Geometry: final body of the model. Coordinates: model frame, mm. Face numbers are marked on the shaded views. Coordinates: 2 decimals unless noted, no trailing zeros. Put each result on its own line as item: value.
```python
from build123d import *

# Parameters (mm, degrees)
F0_R     = 2.75
F1_DEPTH = 21
F1_TAPER = -8
F2_DEPTH = 21.0010001


with BuildPart() as f1:
    # F0 (on Top) → F1 (new body)
    with BuildSketch(Plane.XY):
        with BuildLine():
            ThreePointArc((15.2546531369, -7.0046531369), (21.75, 0), (15.2546531369, 7.0046531369))
            Line((15.2546531369, 7.0046531369), (-14.7453468631, 7.0046531369))
            ThreePointArc((-14.7453468631, 7.0046531369), (-21.75, 0), (-14.7453468631, -7.0046531369))
            Line((-14.7453468631, -7.0046531369), (15.2546531369, -7.0046531369))
        make_face()
        with Locations((-14.7453468631, 0)):
            Circle(F0_R, mode=Mode.SUBTRACT)
        with Locations((15.2546531369, 0)):
            Circle(F0_R, mode=Mode.SUBTRACT)
        with Locations((15.2546531369, 0)):
            Circle(F0_R)
        with Locations((-14.7453468631, 0)):
            Circle(F0_R)
    extrude(amount=-F1_DEPTH, taper=F1_TAPER)

    # F0 (on Top) → F2 (cut, through all)
    with BuildSketch(Plane.XY):
        with Locations((15.2546531369, 0)):
            Circle(F0_R)
        with Locations((-14.7453468631, 0)):
            Circle(F0_R)
    extrude(amount=-F2_DEPTH, mode=Mode.SUBTRACT)


solid = f1.part
```
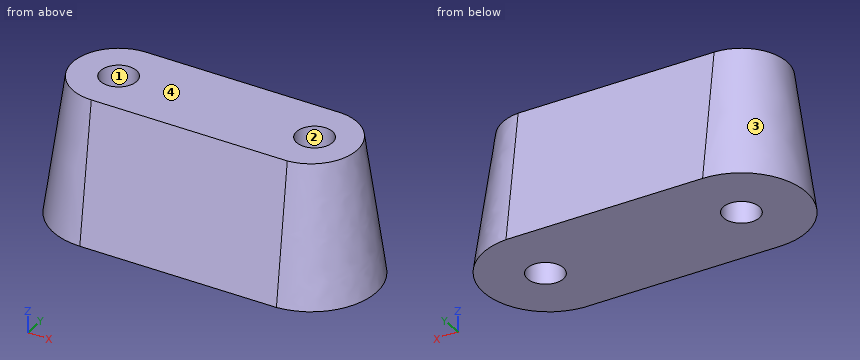
1. Pin query (flat end, axial travel): pin 1 Ø4 at (x, y) = (4.5, 5.5) entering from +Z; pin 2 Ø5 at (x, z) = (-16.5, -4) entering from +Y; pin 3 Ø10 at (y, z) = (3.5, -5.5) entering from -X; pin 4 Ø3 at (x, z) = (-1.5, -8.5) entering from +Y. Return the tip coordinate at first contact, or that it passes through.
Answer below:
pin 1: stops at z = 0
pin 2: stops at y = 7.86
pin 3: stops at x = -23.08
pin 4: stops at y = 8.41
2. Section query A-A (y = 0). Count the separate pieces of the cut face and the enclosed holes in it, then the cut area to 3 significant figures.
Answer below:
separate pieces: 3
enclosed holes: 0
area: 744 mm²
3. Ray query, probe 1 along X at (y, z) = (1.5, -18.25); probe 2 along X at (y, z) = (1.5, -6); probe 3 along Y at (x, z) = (15.5, -17.5). Return the intervals inside material, ascending. Write a range as from..to.
Answer below:
probe 1: x = -24.2..-17.05, -12.44..12.95, 17.56..24.2
probe 2: x = -22.45..-17.05, -12.44..12.95, 17.56..22.45
probe 3: y = -9.45..-2.74, 2.74..9.45
4. Mould query, pull axis X, two halves, no side actions, for the marked faces 1, 2, 3 and 4. Classes: +X half, -X half, draft (parallel to the pull), parting line (faces both ways), or undercut.
Answer below:
face 1: undercut
face 2: undercut
face 3: -X half
face 4: draft
